from build123d import *

# Parameters (mm, degrees)
F2_W     = 238.426886
F2_H     = 151.567214
F3_DEPTH = 3.175
F1_R     = 9.05
F1_R_2   = 9.5
F1_R_3   = 9.7
F1_R_4   = 9.9
F1_R_5   = 10.3
F1_R_6   = 10.5
F1_R_7   = 10.7
F1_R_8   = 10.9
F1_R_9   = 11.1
F1_R_10  = 11.3
F1_R_11  = 10.0965
F0_R     = 7.22
F0_R_2   = 7.4
F0_R_3   = 7.6
F0_R_4   = 7.8
F0_R_5   = 8
F0_R_6   = 8.225
F0_R_7   = 8.45
F0_R_8   = 8.65
F0_R_9   = 8.85
F0_R_10  = 9.1
F4_DEPTH = 25.4


with BuildPart() as f3:
    # F2 (on Front) → F3 (new body)
    with BuildSketch(Plane.XZ):
        with Locations((-13.917122, 0.145737)):
            Rectangle(F2_W, F2_H)
    extrude(amount=F3_DEPTH)

    # F1 (on Front) + F0 (on Front) → F4 (cut)
    with BuildSketch(Plane.XZ):
        with Locations((71.803339, 28.626817)):
            Circle(F1_R)
        with Locations((73.872736, 9.359167)):
            Circle(F1_R_2)
        with Locations((77.738432, -10.366699)):
            Circle(F1_R_3)
        with Locations((74.764473, -31.552281)):
            Circle(F1_R_4)
        with Locations((42.154603, -53.0548)):
            Circle(F1_R_5)
        with Locations((20.467432, -54.267971)):
            Circle(F1_R_6)
        with Locations((-1.80723, -54.662366)):
            Circle(F1_R_7)
        with Locations((-25.024595, -53.251462)):
            Circle(F1_R_8)
        with Locations((-44.686638, -40.878124)):
            Circle(F1_R_9)
        with Locations((-57.200898, -20.724166)):
            Circle(F1_R_10)
        with Locations((62.915616, -48.757901)):
            Circle(F1_R_11)
    with BuildSketch(Plane.XZ):
        with Locations((-65.699088, -2.867658)):
            Circle(F0_R)
        with Locations((-62.893169, 12.845844)):
            Circle(F0_R_2)
        with Locations((-56.141507, 27.393481)):
            Circle(F0_R_3)
        with Locations((-44.119534, 38.547034)):
            Circle(F0_R_4)
        with Locations((-28.320049, 45.309286)):
            Circle(F0_R_5)
        with Locations((-11.58786, 50.566368)):
            Circle(F0_R_6)
        with Locations((5.897778, 54.137864)):
            Circle(F0_R_7)
        with Locations((24.898611, 55.78438)):
            Circle(F0_R_8)
        with Locations((44.18264, 53.365339)):
            Circle(F0_R_9)
        with Locations((62.138096, 45.591767)):
            Circle(F0_R_10)
    extrude(amount=F4_DEPTH, mode=Mode.SUBTRACT)


solid = f3.part
Model file for the job. Use its own axes, mm. Coordinates: 2 decimals unless noted, no trailing zeros. Order: outer loops, then holes, each group sorted by start corner. A loop starts at its lowest first (then second) coordinate and runs counter-clockwise, first axis right, second up. Notation, with made-up numbers: (76, 70.25) -> (105, 70.25) arc R26 cw to (105, 98.25) -> close; hole circle Ø11 at (-10, -33). An arc over 180 degrees is marked (long way). Return JSON: item names as keys, results as strings. Group by question number.
Item 1: Saw through at B-B on x = 43. Write the cut outline in (y, z) (3 decimals).
Item 2: Saw through at A-A on z = -14. Write the cut outline in (x, y) (1 decimal).
Item 3: Pull direction X, two halves, no side cores. Call faces 1 (the cylindrical face through (23.02, -1.57, 47.34)), 2 (the flat face through (-16, -3.175, 1)): pulls with the +X half, pulls with the -X half, needs draft (parallel to the pull), parting line crosses it, or undercut.
Item 4: Wall check: line 1 along X through (y, z) = (-2.4, 9); line 2 along Z through (x, y) = (2.5, -2.95); line 3 along Z through (x, y) = (-41, -1.05). Give the ranges that are in metal, low to high. Write a range as [from, to].
Item 5: Saw through at C-C on y = -1.35. State how many separate pieces and enclosed holes the cut face has, then the cut area to 3 significant figures.
Values found:
{
 "1": {"outline": "(-3.175, -75.638) -> (0, -75.638) -> (0, -63.32) -> (-3.175, -63.32) -> close; (-3.175, -42.79) -> (0, -42.79) -> (0, 44.595) -> (-3.175, 44.595) -> close; (-3.175, 62.136) -> (0, 62.136) -> (0, 75.929) -> (-3.175, 75.929) -> close"},
 "2": {"outline": "(-133.1, -3.2) -> (-66.3, -3.2) -> (-66.3, 0) -> (-133.1, 0) -> close; (-48.1, -3.2) -> (68.7, -3.2) -> (68.7, 0) -> (-48.1, 0) -> close; (86.7, -3.2) -> (105.3, -3.2) -> (105.3, 0) -> (86.7, 0) -> close"},
 "3": {"face 1": "undercut", "face 2": "needs draft"},
 "4": {"line 1": "x = [-133.13, -69.22], [-56.57, 64.38], [83.37, 105.3]", "line 2": "z = [-75.64, -64.46], [-44.87, 46.4], [61.87, 75.93]", "line 3": "z = [-75.64, -51.35], [-30.41, 31.4], [45.7, 75.93]"},
 "5": {"separate pieces": "1", "enclosed holes": "21", "area": "30,400 mm2"}
}
